Build history of the part. All positions in model axes, mm. A direction names the side the tool comes from. Give positions to 0.01 mm unless a question says otherwise; leave off trailing zeros. Order: outer loops, then holes, each group sorted by start corner. A loop starts at its lowest first (then second) coordinate and runs counter-clockwise, first axis right, second up. Notation, with made-up numbers: (87.5, 69.5) - (101.5, 69.5) arc R24 ccw to (101.5, 89.5) - close; hole circle Ø3 at (-12.5, 77.5). An arc over 180 degrees is marked (long way). Use a Markdown table: item, result. Add a question column.
(1) Which spindle directions (+Z, -Z, +X, -X, +Y, -Y) get a long thin tool onto all of the face, cutting with end or side? Do faces 1 (the face through (165.4, -0.5, 8.5)), 2 (the face through (160.954, -1.2, 12.1)), 3 (the face through (163.445, -2.26, 2.261)). Say none if no direction does.
(2) Flat gauge pins, fed straight in: pin 1 (3 mm diameter, centred on x = 164.5, z = 18, fed in from -Y); pin 2 (2.5 mm diameter, centred on x = 165.96, z = 4.25, fed in from +Y). Where does each tip first touch, or does it go through?
(3) Slice it at C-C (x = 167). Write the cut outline in (y, z).
(4) Wall check: line 1 (X direction, y = -1, z = 19.75); line 2 (Z direction, x = 167.5, y = -0.45); line 3 (Y direction, x = 168.25, z = 10.5). Give the ranges that are in metal, low to high.
(5) Slice it at D-D (z = 9.75). Write the cut outline in (x, y), then the cut area to 3 significant figures.
(6) Mould opens along Z. For faces 4 (the face through (166, -1, 22)), 5 (the face through (162.981, -2, 20)), 6 (the face through (169.954, -1.5, 12.1)) say: +Z half, -Z half, draft (parallel to the pull), parting line (faces both ways), or undercut.
(7) Slice it at A-A (y = -0.7). Write the cut outline in (x, z).
(8) Slice it at B-B (z = 19.75). Write the cut outline in (x, y), then the cut area to 3 significant figures.
from build123d import *

# Parameters (mm, degrees)
CROQUIS1_W              = 9
CROQUIS1_H              = 20
CROQUIS1_R              = 1.7
SALIENTE_EXTRUIR1_DEPTH = 3
CORTAR_EXTRUIR2_DEPTH   = 1.5
CORTAR_EXTRUIR3_REACH   = 25.958
CROQUIS3_W              = 7
CROQUIS3_H              = 1
REDONDEO1_R             = 1


with BuildPart() as part:
    # Croquis1 → Saliente-Extruir1 (new body)
    with BuildSketch(Plane(origin=(0, 0, 0), x_dir=(1, 0, 0), z_dir=(0, 1, 0))):
        with Locations((165.454426616, -12)):
            Rectangle(CROQUIS1_W, CROQUIS1_H)
        with Locations(Location((165.962302832, -4.25, 0), (0, 0, 270))):
            Circle(CROQUIS1_R, mode=Mode.SUBTRACT)
        with Locations(Location((165.962302832, -19.75, 0), (0, 0, 270))):
            Circle(CROQUIS1_R, mode=Mode.SUBTRACT)
    extrude(amount=-SALIENTE_EXTRUIR1_DEPTH)

    # Croquis2 → Cortar-Extruir2 (cut)
    with BuildSketch(Plane.XZ.offset(3)):
        Polygon((168.943819954, 21.471379713), (165.962302832, 23.192759426), (162.98078571, 21.471379713), (162.98078571, 18.028620287), (165.962302832, 16.307240574), (168.943819954, 18.028620287), align=None)
        Polygon((168.943819954, 5.971379713), (168.943819954, 2.528620287), (165.962302832, 0.807240574), (162.98078571, 2.528620287), (162.98078571, 5.971379713), (165.962302832, 7.692759426), align=None)
    extrude(amount=-CORTAR_EXTRUIR2_DEPTH, mode=Mode.SUBTRACT)

    # Croquis3 → Cortar-Extruir3 (cut, up to next)
    with BuildSketch(Plane.ZY.offset(-160.954426616), mode=Mode.PRIVATE) as cortar_extruir3_sk1:
        with Locations((12, -0.5)):
            Rectangle(CROQUIS3_W, CROQUIS3_H)
    cortar_extruir3_tool1 = extrude(cortar_extruir3_sk1.sketch, amount=-CORTAR_EXTRUIR3_REACH, mode=Mode.PRIVATE) & part.part
    add(cortar_extruir3_tool1.solids().sort_by_distance((160.954427, -0.5, 12))[0], mode=Mode.SUBTRACT)

    # Redondeo1
    redondeo1_edges = [part.edges().sort_by_distance(p)[0] for p in [
        (160.954426616, -3, 12),
        (160.954426616, -1.5, 2),
        (160.954426616, -1.5, 22),
    ]]
    fillet(redondeo1_edges, radius=REDONDEO1_R)


solid = part.part
Solution:
| question | item | result |
|---|---|---|
| 1 | face 1 | +X, -X, +Y |
| 1 | face 2 | +Z, -Z, -X, +Y, -Y |
| 1 | face 3 | -Y |
| 2 | pin 1 | y = -3 |
| 2 | pin 2 | through |
| 3 | outline | (-3, 7.09) - (-1.5, 7.09) - (-1.5, 5.6) - (0, 5.6) - (0, 8.5) - (-1, 8.5) - (-1, 15.5) - (0, 15.5) - (0, 18.4) - (-1.5, 18.4) - (-1.5, 16.91) - (-3, 16.91) - close; (-1.5, 2) - (0, 2) - (0, 2.9) - (-1.5, 2.9) - close; (-1.5, 21.1) - (0, 21.1) - (0, 22) - (-1.5, 22) - close |
| 4 | line 1 | 160.95 to 164.26, 167.66 to 169.95 |
| 4 | line 2 | 2 to 3.53, 4.97 to 8.5, 15.5 to 19.03, 20.47 to 22 |
| 4 | line 3 | -3 to -1 |
| 5 | outline | (160.95, -2) arc R1 ccw to (161.95, -3) - (169.95, -3) - (169.95, -1) - (160.95, -1) - close |
| 5 | area | 17.8 mm2 |
| 6 | face 4 | +Z half |
| 6 | face 5 | undercut |
| 6 | face 6 | draft |
| 7 | outline | (160.95, 3) arc R1 ccw to (161.95, 2) - (169.95, 2) - (169.95, 8.5) - (160.95, 8.5) - close; (160.95, 15.5) - (169.95, 15.5) - (169.95, 22) - (161.95, 22) arc R1 ccw to (160.95, 21) - close; hole circle Ø3.4 at (165.96, 4.25); hole circle Ø3.4 at (165.96, 19.75) |
| 8 | outline | (160.95, -2) arc R1 ccw to (161.95, -3) - (162.98, -3) - (162.98, -1.5) - (164.26, -1.5) - (164.26, 0) - (160.95, 0) - close; (167.66, -1.5) - (168.94, -1.5) - (168.94, -3) - (169.95, -3) - (169.95, 0) - (167.66, 0) - close |
| 8 | area | 12.7 mm2 |
